Check sheet for the drawn part. Datum: minimum x, y, z corner. Units: mm. Give positions to 0.01 mm unless a question says otherwise; leave off trailing zeros. Loops run counter-clockwise (first coordinate to the right, second up) from the corner with the lowest first, then second, coordinate; pieces in that order, holes last. Notation, with made-up numbers: (-15, 78.5) - (18, 78.5) arc R22 ccw to (18, 94.5) - close; hole circle Ø9 at (40.5, 25.5). An arc over 180 degrees is marked (long way). Use a Markdown table: item, result. Add a question column.
1. Material ranges on L1, parallel to Y at x = 24.55, z = 18; L2, parallel to Y at x = 2.75, z = 24; L3, parallel to Y at x = 14.25, z = 3.5 (1 decimal), recorded low to high.
2. Cross-section at A-A on z = 18. Enter the section's corners in (x, y).
3. Cross-section at C-C on z = 10. Enter the section's corners in (x, y).
4. Draft check along Y on the marked faces 1, 2, 3 and 4. Enter one of: pulls with the +Y half, pulls with the -Y half, needs draft (parallel to the pull), parting line crosses it, or undercut.
5. Cross-section at B-B on x = 11.5. Enter the section's corners in (y, z), and give its area (3 significant figures).
6. Depth check by flat-ended pin: P1, Ø2, axis at x = 5.5, y = 35, coming from the -Z side; P2, Ø2.5, axis at x = 20.5, y = 5, coming from the -Z side; P3, Ø2, axis at y = 12, z = 30.5, coming from the +X side. Enter the tip coordinate at first touch or a pass-through.
7. Cross-section at D-D on z = 40. Enter the section's corners in (x, y), and give its area (3 significant figures).
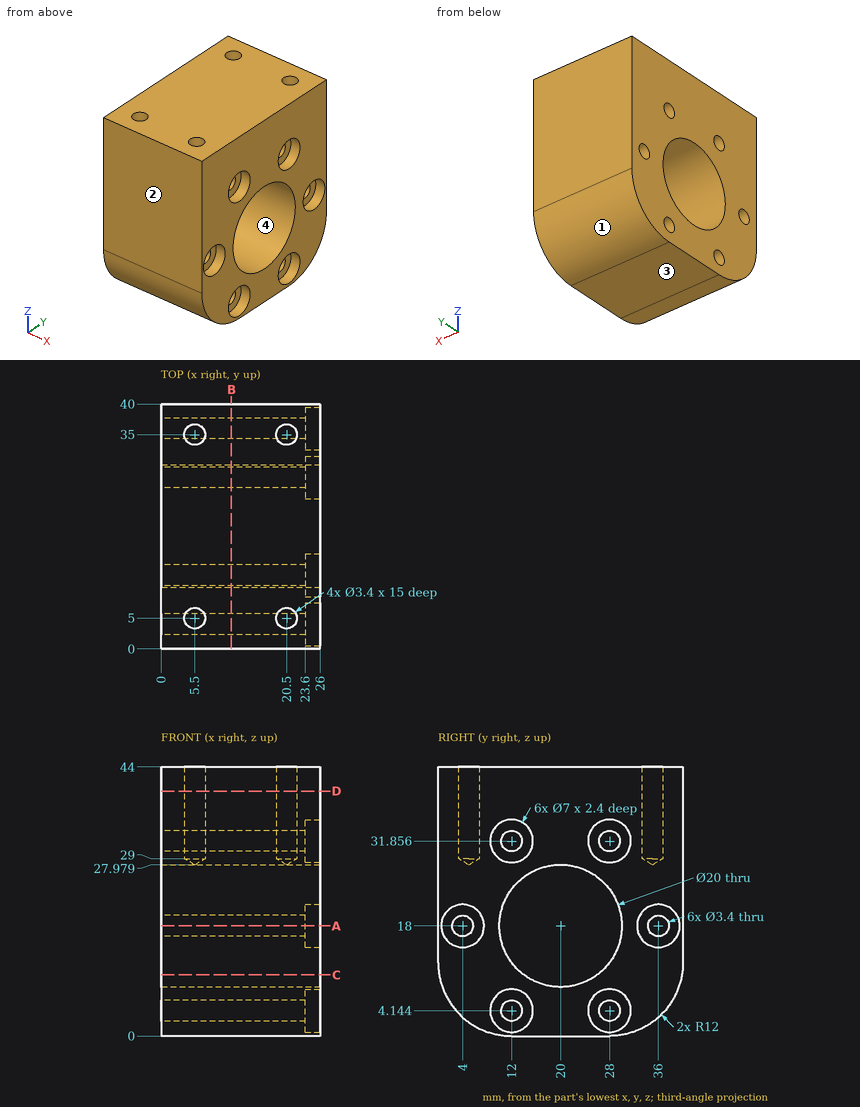
Values found:
| question | item | result |
|---|---|---|
| 1 | L1 | y = 0 to 0.5, 7.5 to 10, 30 to 32.5, 39.5 to 40 |
| 1 | L2 | y = 0 to 12, 28 to 40 |
| 1 | L3 | y = 3.5 to 10.4, 13.6 to 26.4, 29.6 to 36.5 |
| 2 | outline | (0, 0) - (26, 0) - (26, 0.5) - (23.6, 0.5) - (23.6, 2.3) - (0, 2.3) - close; (0, 5.7) - (23.6, 5.7) - (23.6, 7.5) - (26, 7.5) - (26, 10) - (0, 10) - close; (0, 30) - (26, 30) - (26, 32.5) - (23.6, 32.5) - (23.6, 34.3) - (0, 34.3) - close; (0, 37.7) - (23.6, 37.7) - (23.6, 39.5) - (26, 39.5) - (26, 40) - (0, 40) - close |
| 3 | outline | (0, 0.17) - (26, 0.17) - (26, 14) - (0, 14) - close; (0, 26) - (26, 26) - (26, 39.83) - (0, 39.83) - close |
| 4 | face 1 | pulls with the +Y half |
| 4 | face 2 | pulls with the -Y half |
| 4 | face 3 | needs draft |
| 4 | face 4 | undercut |
| 5 | outline | (0, 12) arc R12 ccw to (12, 0) - (28, 0) arc R12 ccw to (40, 12) - (40, 44) - (0, 44) - close; hole circle Ø3.4 at (4, 18); hole circle Ø20 at (20, 18); hole circle Ø3.4 at (12, 4.14); hole circle Ø3.4 at (12, 31.86); hole circle Ø3.4 at (28, 4.14); hole circle Ø3.4 at (28, 31.86); hole circle Ø3.4 at (36, 18) |
| 5 | area | 1,330 mm2 |
| 6 | P1 | stops at z = 1.61 |
| 6 | P2 | stops at z = 1.47 |
| 6 | P3 | stops at x = 23.6 |
| 7 | outline | (0, 0) - (26, 0) - (26, 40) - (0, 40) - close; hole circle Ø3.4 at (5.5, 5); hole circle Ø3.4 at (5.5, 35); hole circle Ø3.4 at (20.5, 5); hole circle Ø3.4 at (20.5, 35) |
| 7 | area | 1,000 mm2 |
